```python
from build123d import *

# Parameters (mm, degrees)
F0_W     = 180
F0_H     = 105
F0_W_2   = 230
F0_H_2   = 55
F0_W_3   = 170
F0_H_3   = 20
F1_DEPTH = 10
F2_R     = 1


with BuildPart() as f1:
    # F0 (on Top) → F1 (new body)
    with BuildSketch(Plane.XY):
        Polygon((85, -129.952139), (115, 115.047861), (-115, 115.047861), (-85, -129.952139), (-85, -109.952139), (85, -109.952139), align=None)
        with Locations((0, 56.453109)):
            Rectangle(F0_W, F0_H, mode=Mode.SUBTRACT)
        with Locations((0, 142.547861)):
            Rectangle(F0_W_2, F0_H_2)
        with Locations((0, -119.952139)):
            Rectangle(F0_W_3, F0_H_3)
    extrude(amount=F1_DEPTH)

    # F2
    f2_edges = [f1.edges().sort_by_distance(p)[0] for p in [
        (0, 108.953109, 0),
        (90, 56.453109, 10),
        (0, 3.953109, 10),
        (-90, 56.453109, 10),
        (0, 3.953109, 0),
        (-90, 56.453109, 0),
        (0, 108.953109, 10),
        (90, 56.453109, 0),
    ]]
    fillet(f2_edges, radius=F2_R)


solid = f1.part
```
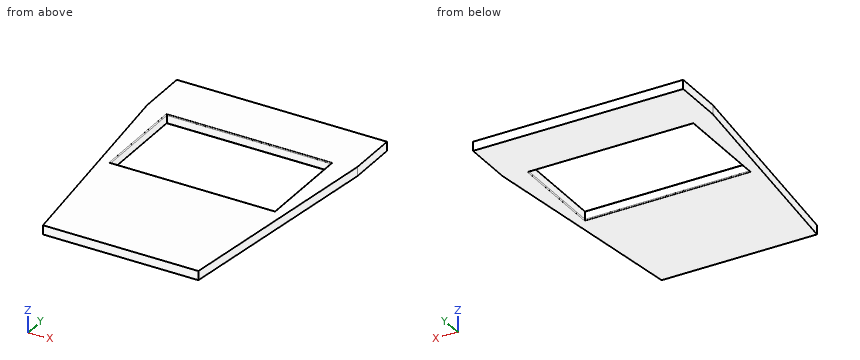
Verification items for the finished model (mm, model axes). Coordinates: 2 decimals unless noted, no trailing zeros. Order: outer loops, then holes, each group sorted by start corner. A loop starts at its lowest first (then second) coordinate and runs counter-clockwise, first axis right, second up. Notation, with made-up numbers: (-25, -3.5) -> (0, -3.5) arc R29 cw to (0, 21.5) -> close; hole circle Ø11 at (22, 57). An arc over 180 degrees is marked (long way). Answer as CSV lines item,"result". Start each with the question number.
1) Gauge pin test, flat ends, axial feed: pin 1 Ø2.5 at (y, z) = (69.5, 6) entering from -X; pin 2 Ø5 at (y, z) = (-81.5, 3.5) entering from -X; pin 3 Ø1.5 at (y, z) = (103.5, 2.5) entering from -X. Record the tip position at first contact, or that the pin passes through.
2) Cross-section at B-B, the plane z = 4. Record the boundary of the cut face in (x, y), then the cut area to 4 significant figures.
3) Cross-section at D-D, the plane y = -29. Record the boundary of the cut face in (x, z).
4) Cross-section at A-A, the plane x = -6. Record the boundary of the cut face in (y, z), then the cut area to 3 significant figures.
5) Cross-section at C-C, the plane y = 81.5. Record the boundary of the cut face in (x, z).
6) Material ranges on L1, parallel to Y at x = 83.5, z = 6; L2, parallel to X at y = 101, z = 1.5; L3, parallel to X at y = 18, z = 5.5, recorded low to high. Write a range as [from, to].
Conclusion:
1,pin 1,"stops at x = -109.58"
1,pin 2,"stops at x = -91.24"
1,pin 3,"stops at x = -113.68"
2,outline,"(-115, 115.05) -> (-85, -129.95) -> (85, -129.95) -> (115, 115.05) -> (115, 170.05) -> (-115, 170.05) -> close; hole (-90, 3.95) -> (90, 3.95) -> (90, 108.95) -> (-90, 108.95) -> close"
2,area,"42,750 mm²"
3,outline,"(-97.36, 0) -> (97.36, 0) -> (97.36, 10) -> (-97.36, 10) -> close"
4,outline,"(-129.95, 0) -> (2.95, 0) arc R1 ccw to (3.95, 1) -> (3.95, 9) arc R1 ccw to (2.95, 10) -> (-129.95, 10) -> close; (108.95, 1) arc R1 ccw to (109.95, 0) -> (170.05, 0) -> (170.05, 10) -> (109.95, 10) arc R1 ccw to (108.95, 9) -> close"
4,area,"1,950 mm²"
5,outline,"(-110.89, 0) -> (-91, 0) arc R1 ccw to (-90, 1) -> (-90, 9) arc R1 ccw to (-91, 10) -> (-110.89, 10) -> close; (90, 1) arc R1 ccw to (91, 0) -> (110.89, 0) -> (110.89, 10) -> (91, 10) arc R1 ccw to (90, 9) -> close"
6,L1,"y = [-129.95, 3.95], [108.95, 170.05]"
6,L2,"x = [-113.28, -90], [90, 113.28]"
6,L3,"x = [-103.12, -90], [90, 103.12]"
